from build123d import *

# Parameters (mm, degrees)
SKETCH1_R           = 2.1
BOSS_EXTRUDE1_DEPTH = 463


with BuildPart() as part:
    # Sketch1 → Boss-Extrude1 (new body)
    with BuildSketch(Plane.XY):
        with BuildLine():
            Line((0, 1), (0, 5.36))
            Line((0, 5.36), (1.8, 7.16))
            Line((1.8, 7.16), (1.8, 4.500660172))
            Line((1.8, 4.500660172), (3.44, 4.500660172))
            Line((3.44, 4.500660172), (6.099339828, 7.16))
            Line((6.099339828, 7.16), (6.099339828, 12.84))
            Line((6.099339828, 12.84), (3.44, 15.499339828))
            Line((3.44, 15.499339828), (1.8, 15.499339828))
            Line((1.8, 15.499339828), (1.8, 12.84))
            Line((1.8, 12.84), (0, 14.64))
            Line((0, 14.64), (0, 19))
            ThreePointArc((0, 19), (0.292893219, 19.707106781), (1, 20))
            Line((1, 20), (5.36, 20))
            Line((5.36, 20), (7.16, 18.2))
            Line((7.16, 18.2), (4.500660172, 18.2))
            Line((4.500660172, 18.2), (4.500660172, 16.56))
            Line((4.500660172, 16.56), (7.16, 13.900660172))
            Line((7.16, 13.900660172), (12.84, 13.900660172))
            Line((12.84, 13.900660172), (15.464579042, 16.525239214))
            Line((15.464579042, 16.525239214), (15.464579042, 18.165239214))
            Line((15.464579042, 18.165239214), (12.84, 18.2))
            Line((12.84, 18.2), (14.64, 20))
            Line((14.64, 20), (19, 20))
            ThreePointArc((19, 20), (19.707106781, 19.707106781), (20, 19))
            Line((20, 19), (20, 14.674581351))
            Line((20, 14.674581351), (18.155899385, 12.84))
            Line((18.155899385, 12.84), (18.155899385, 15.455239214))
            Line((18.155899385, 15.455239214), (16.515899385, 15.455239214))
            Line((16.515899385, 15.455239214), (13.900660172, 12.84))
            Line((13.900660172, 12.84), (13.900660172, 7.16))
            Line((13.900660172, 7.16), (16.56, 4.500660172))
            Line((16.56, 4.500660172), (18.2, 4.500660172))
            Line((18.2, 4.500660172), (18.2, 7.16))
            Line((18.2, 7.16), (20, 5.36))
            Line((20, 5.36), (20, 1))
            ThreePointArc((20, 1), (19.707106781, 0.292893219), (19, 0))
            Line((19, 0), (14.64, 0))
            Line((14.64, 0), (12.84, 1.8))
            Line((12.84, 1.8), (15.499339828, 1.8))
            Line((15.499339828, 1.8), (15.499339828, 3.44))
            Line((15.499339828, 3.44), (12.84, 6.099339828))
            Line((12.84, 6.099339828), (7.16, 6.099339828))
            Line((7.16, 6.099339828), (4.500660172, 3.44))
            Line((4.500660172, 3.44), (4.500660172, 1.8))
            Line((4.500660172, 1.8), (7.16, 1.8))
            Line((7.16, 1.8), (5.36, 0))
            Line((5.36, 0), (1, 0))
            ThreePointArc((1, 0), (0.292893219, 0.292893219), (0, 1))
        make_face()
        with Locations((10.02040103, 9.97959897)):
            Circle(SKETCH1_R, mode=Mode.SUBTRACT)
        Polygon((16.534579042, 18.2), (16.534579042, 17.576559557), (17.585899385, 16.525239214), (18.2, 16.525239214), (18.2, 18.2), align=None, mode=Mode.SUBTRACT)
        Polygon((18.2, 1.75919794), (18.2, 3.433958726), (17.585899385, 3.433958726), (16.534579042, 2.382638382), (16.534579042, 1.75919794), align=None, mode=Mode.SUBTRACT)
        Polygon((2.454902675, 16.525239214), (1.84080206, 16.525239214), (1.84080206, 18.2), (3.506223018, 18.2), (3.506223018, 17.576559557), align=None, mode=Mode.SUBTRACT)
        Polygon((3.506223018, 1.75919794), (1.84080206, 1.75919794), (1.84080206, 3.433958726), (2.454902675, 3.433958726), (3.506223018, 2.382638382), align=None, mode=Mode.SUBTRACT)
    extrude(amount=-BOSS_EXTRUDE1_DEPTH)


solid = part.part
Work out the finished part from the listing and answer in its coordinate system (mm). Coordinates: 2 decimals unless noted, no trailing zeros.
1. Flat-ended cylindrical pins translate along their axes: pin 1 (1.7 mm diameter, centred on y = 11, z = -286.5, fed in from +X); pin 2 (6 mm diameter, centred on y = 9, z = -259.5, fed in from -X); pin 3 (1.7 mm diameter, centred on x = 9, z = -205, fed in from -Y). Find the tip coordinate at first contact, or state that the pin passes through.
Results list:
pin 1: stops at x = 13.9
pin 2: stops at x = 0.64
pin 3: stops at y = 6.1
2. The part is cut by section A-A, the plane z = -132. State how many separate pieces and enclosed holes the cut face has, and give its area (3 significant figures).
Results list:
separate pieces: 1
enclosed holes: 5
area: 162 mm2
3. Consider line 1 along Y through (x, z) = (17.5, -413.5); line 2 along X through (y, z) = (2.25, -38); line 3 along X through (y, z) = (6.5, -323.5). Determine where each line is inside the solid, lowest interval first.
Results list:
line 1: y = 0 to 1.76, 3.35 to 4.5, 15.46 to 16.61, 18.2 to 20
line 2: x = 0 to 1.84, 3.51 to 4.5, 15.5 to 16.53, 18.2 to 20
line 3: x = 1.14 to 1.8, 5.44 to 14.56, 18.2 to 18.86
